The model under review builds one solid part; all positions refer to its coordinate system, in mm. A direction names the side the tool comes from. Round coordinates to 2 decimals unless told otherwise and drop trailing zeros. Order: outer loops, then holes, each group sorted by start corner. A loop starts at its lowest first (then second) coordinate and runs counter-clockwise, first axis right, second up.
1) Machinability: for faces 5 (the face through (29.58, 37.966, -10.479)), 6 (the face through (30, 13, -5)), 7 (the face through (23, -44, -5)), 8 (the face through (30, 45, -5)), which of the approach directions +Z, -Z, +X, -X, +Y, -Y give a long, thin tool a straight path to every point of the face, cutting with its end or side? Answer none if there is none.
2) Consider section B-B (y = -8). Give the boundary of the cut face in (x, z), then the cut area to 3 significant figures.
3) Clearance check with flat-ended pins moving along their axes: P1, Ø3.5, axis at x = 39, z = -14, coming from the +Y side; P2, Ø3.5, axis at x = 45, z = -11.5, coming from the -Y side; P3, Ø5, axis at x = 26.5, y = 44.5, coming from the -Z side. State where each tip first meets the part, or that it passes through.
4) To check wall thickness, follow L1, parallel to Y at x = 29, z = -11; L2, parallel to Y at x = 43, z = -8.25; L3, parallel to Y at x = 32.5, z = -6. State the ranges of each line that lie inside material, in increasing order.
5) Consider section A-A (x = 30). Give the boundary of the cut face in (y, z), then the cut area to 3 significant figures.
6) Mouldability with a two-part tool opening along Y and no side actions: class faces 1 (the face through (30, 34, -17)), 2 (the face through (30, 40, -11)), 3 (the face through (30, 28, -11)), 4 (the face through (29.6, -10.4, -7.8)) as pulls with the +Y half, pulls with the -Y half, needs draft (parallel to the pull), parting line crosses it, or undercut.
7) Consider section D-D (z = -1.75). Give the boundary of the cut face in (x, y), then the cut area to 3 significant figures.
8) Consider section C-C (x = 12). Give the boundary of the cut face in (y, z).
from build123d import *

# Parameters (mm, degrees)
SKETCH_1_R          = 4
EXTRUDE_1_DEPTH     = 60
SKETCH_2_R          = 15
CUT_EXTRUDE_1_DEPTH = 60


with BuildPart() as part:
    # 草图1 → 凸台-拉伸1 (new body)
    with BuildSketch(Plane(origin=(0, 0, 0), x_dir=(0, 0, -1), z_dir=(1, 0, 0))):
        Polygon((5, -2), (5, 28), (17, 28), (17, 40), (5, 40), (5, 50), (-5, 50), (-5, -50), (5, -50), (5, -14), (17, -14), (17, -2), align=None)
        with Locations((11, 34)):
            Circle(SKETCH_1_R, mode=Mode.SUBTRACT)
        with Locations((11, -8)):
            Circle(SKETCH_1_R, mode=Mode.SUBTRACT)
    extrude(amount=EXTRUDE_1_DEPTH)

    # 草图2 → 切除-拉伸1 (cut)
    with BuildSketch(Plane.XY.offset(5)):
        with Locations((30, -30)):
            Circle(SKETCH_2_R)
    extrude(amount=-CUT_EXTRUDE_1_DEPTH, mode=Mode.SUBTRACT)


solid = part.part
Answer below:
1. face 5: +X, -X
1. face 6: -Z, +X, -X
1. face 7: -Z, +X, -X, -Y
1. face 8: -Z, +X, -X, +Y
2. outline: (0, -17) - (60, -17) - (60, -15) - (0, -15) - close; (0, -7) - (60, -7) - (60, 5) - (0, 5) - close
2. area: 840 mm2
3. P1: stops at y = 40
3. P2: stops at y = -14
3. P3: stops at z = -5
4. L1: y = -14 to -12, -4 to -2, 28 to 30, 38 to 40
4. L2: y = -14 to -10.9, -5.1 to -2, 28 to 31.1, 36.9 to 40
4. L3: y = -14 to -2, 28 to 40
5. outline: (-50, -5) - (-45, -5) - (-45, 5) - (-50, 5) - close; (-15, -5) - (-14, -5) - (-14, -17) - (-2, -17) - (-2, -5) - (28, -5) - (28, -17) - (40, -17) - (40, -5) - (50, -5) - (50, 5) - (-15, 5) - close; hole circle Ø8 at (-8, -11); hole circle Ø8 at (34, -11)
5. area: 887 mm2
6. face 1: needs draft
6. face 2: pulls with the +Y half
6. face 3: undercut
6. face 4: undercut
7. outline: (0, -50) - (60, -50) - (60, 50) - (0, 50) - close; hole circle Ø30 at (30, -30)
7. area: 5,290 mm2
8. outline: (-50, -5) - (-14, -5) - (-14, -17) - (-2, -17) - (-2, -5) - (28, -5) - (28, -17) - (40, -17) - (40, -5) - (50, -5) - (50, 5) - (-50, 5) - close; hole circle Ø8 at (-8, -11); hole circle Ø8 at (34, -11)
